Answer from the drawing. Dimensions are ordinates in mm from the lowest x, y and z of the part. Coordinates: 2 decimals unless noted, no trailing zeros. Write each loop counter-clockwise with the first axis right and the second up, starting at its lowest first coordinate (ties: lowest second). Pieces come first, ordered by that corner, then holes. Notation, with made-up numbers: (25.25, 21.25) - (36.25, 21.25) arc R14 ccw to (36.25, 48.25) - close; hole circle Ø9 at (48.5, 30.25). An arc over 180 degrees is marked (long way). Answer as a JSON object with one key per item and string values. Group by question number.
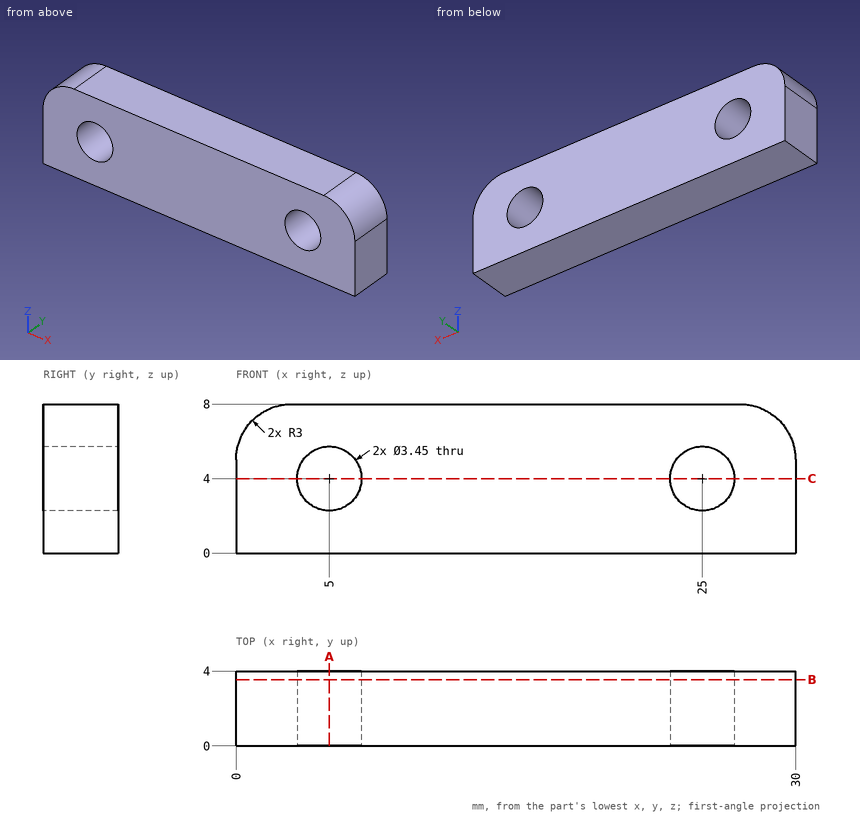
Q1. Consider L1, parallel to X at y = 2.35, z = 4 (3 decimals); L2, parallel to X at y = 2.6, z = 5.5; L3, parallel to Z at x = 6, y = 0.5. Determine where each line is inside the solid, lowest interval first. Write a range as from..to.
Q2. Section C-C on z = 4 is taken. Determine the outline of the cut face in (x, y) (3 decimals), plus the area to 3 significant figures.
Q3. Section B-B on y = 3.55 is taken. Determine the outline of the cut face in (x, z) (3 decimals), plus the area to 3 significant figures.
Q4. Section A-A on x = 5 is taken. Determine the outline of the cut face in (y, z) (3 decimals).
Numbers:
{
 "1": {"L1": "x = 0..3.275, 6.725..23.275, 26.725..30", "L2": "x = 0.04..4.15, 5.85..24.15, 25.85..29.96", "L3": "z = 0..2.59, 5.41..8"},
 "2": {"outline": "(0, 0) - (3.275, 0) - (3.275, 4) - (0, 4) - close; (6.725, 0) - (23.275, 0) - (23.275, 4) - (6.725, 4) - close; (26.725, 0) - (30, 0) - (30, 4) - (26.725, 4) - close", "area": "92.4 mm²"},
 "3": {"outline": "(0, 0) - (30, 0) - (30, 5) arc R3 ccw to (27, 8) - (3, 8) arc R3 ccw to (0, 5) - close; hole circle Ø3.45 at (5, 4); hole circle Ø3.45 at (25, 4)", "area": "217 mm²"},
 "4": {"outline": "(0, 0) - (4, 0) - (4, 2.275) - (0, 2.275) - close; (0, 5.725) - (4, 5.725) - (4, 8) - (0, 8) - close"}
}
